from build123d import *

# Parameters (mm, degrees)
F0_R     = 6
F1_DEPTH = 10
F2_R     = 10
F3_DEPTH = 8


with BuildPart() as f1:
    # F0 (on Top) → F1 (new body)
    with BuildSketch(Plane.XY):
        with BuildLine():
            ThreePointArc((-2.287583, -36.367918), (14.118454, -23.224109), (34.477123, -17.985565))
            ThreePointArc((34.477123, -17.985565), (51.756399, 0), (34.477123, 17.985565))
            ThreePointArc((34.477123, 17.985565), (14.118454, 23.224109), (-2.287583, 36.367918))
            ThreePointArc((-2.287583, 36.367918), (-21.61854, 42.178767), (-34.190148, 26.386157))
            Line((-34.190148, 26.386157), (-34.190148, 23.613843))
            Line((-34.190148, 23.613843), (-34.190148, -23.613843))
            Line((-34.190148, -23.613843), (-34.190148, -26.386157))
            ThreePointArc((-34.190148, -26.386157), (-21.61854, -42.178767), (-2.287583, -36.367918))
        make_face()
        with Locations((-16.243601, -25)):
            Circle(F0_R, mode=Mode.SUBTRACT)
        with Locations((33.756399, 0)):
            Circle(F0_R, mode=Mode.SUBTRACT)
        with Locations((-16.243601, 25)):
            Circle(F0_R, mode=Mode.SUBTRACT)
    extrude(amount=F1_DEPTH)

    # F2 (on Front) → F3 (join, symmetric)
    with BuildSketch(Plane.XZ):
        with BuildLine():
            Line((-75.522877, 0), (18.498397, 0))
            Line((18.498397, 0), (18.498397, 10))
            ThreePointArc((18.498397, 10), (-24.010105, 17.449895), (-61.451666, 38.911565))
            ThreePointArc((-61.451666, 38.911565), (-96.211695, 29.481496), (-75.522877, 0))
        make_face()
        with Locations((-75.522877, 22)):
            Circle(F2_R, mode=Mode.SUBTRACT)
    extrude(amount=F3_DEPTH, both=True)


solid = f1.part
Input: part model. Units: mm. Frame: model coordinates. A direction names the side the tool comes from. Give positions to 0.01 mm unless a question says otherwise; leave off trailing zeros. Order: outer loops, then holes, each group sorted by start corner. A loop starts at its lowest first (then second) coordinate and runs counter-clockwise, first axis right, second up. Notation, with made-up numbers: (34, -5) - (52, -5) arc R16 ccw to (52, 9) - close; hole circle Ø6 at (-37, -36.75). An arc over 180 degrees is marked (long way). Answer as a JSON object with one key per item and string values. Group by question number.
Q1. Line query: probe 1 along Z at (x, y) = (-76, 6.5); probe 2 along Y at (x, z) = (-49, 14.5); probe 3 along X at (y, z) = (-4, 3.5). Output: solid intervals per line, ascending.
Q2. Mould query, pull axis Y, two halves, no side actions, for faces 1 (the face through (-13, -1, 0)), 2 (the face through (-21.9, -42.09, 4.93)), 3 (the face through (14.384, 23.092, 4.93)), 4 (the face through (-10.7, -27.3, 4.9)). Classes: pulls with the +Y half, pulls with the -Y half, needs draft (parallel to the pull), parting line crosses it, or undercut.
Q3. First-contact query: pin 1 Ø12 at (x, z) = (-72.5, 15.5) entering from +Y; pin 2 Ø6 at (y, z) = (-2.5, 25.5) entering from +X; pin 3 Ø7 at (x, y) = (-16.24, -25) entering from +Z; pin 4 Ø19 at (x, y) = (33.76, 0) entering from +Z. Flat tips, straight axial feed; report the tip coordinate or a pass-through.
Q4. Set-up query: faces 5 (the face through (-34.19, 17, 5)), 6 (the face through (-70.1, 0.1, 30.4)), 7 (the face through (-34.19, -17, 5)). Return all of +Z, -Z, +X, -X, +Y, -Y with unobstructed straight access to the full face (end or side cutting, diameter ignored); none if empty.
Q5. Cut plane A-A, the plane y = 0. Output: boundary loops of the cut face in (x, z).
Q6. Cut plane D-D, the plane y = -28.5. Output: boundary loops of the cut face in (x, z).
Q7. Cut plane C-C, the plane z = 17. Output: boundary loops of the cut face in (x, y).
Q8. Cut plane B-B, the plane x = -18. Output: boundary loops of the cut face in (y, z), then the cut area to 3 significant figures.
Results:
{
 "1": {"probe 1": "0.01 to 12.01, 31.99 to 43.99", "probe 2": "-8 to 8", "probe 3": "-87.43 to 29.28, 38.23 to 51.31"},
 "2": {"face 1": "needs draft", "face 2": "pulls with the -Y half", "face 3": "pulls with the +Y half", "face 4": "undercut"},
 "3": {"pin 1": "y = 8", "pin 2": "x = -35.99", "pin 3": "through", "pin 4": "z = 10"},
 "4": {"face 5": "+Z, -Z, -X, +Y", "face 6": "+Y, -Y", "face 7": "+Z, -Z, -X, -Y"},
 "5": {"outline": "(-75.52, 0) - (27.76, 0) - (27.76, 10) - (18.5, 10) arc R125 cw to (-61.45, 38.91) arc R22 ccw (long way) to start; (39.76, 0) - (51.76, 0) - (51.76, 10) - (39.76, 10) - close; hole circle Ø20 at (-75.52, 22)"},
 "6": {"outline": "(-33.9, 0) - (-21.12, 0) - (-21.12, 10) - (-33.9, 10) - close; (-11.37, 0) - (5.75, 0) - (5.75, 10) - (-11.37, 10) - close"},
 "7": {"outline": "(-96.95, -8) - (-84.18, -8) - (-84.18, 8) - (-96.95, 8) - close; (-66.86, -8) - (-22.74, -8) - (-22.74, 8) - (-66.86, 8) - close"},
 "8": {"outline": "(-42.91, 0) - (-30.74, 0) - (-30.74, 10) - (-42.91, 10) - close; (-19.26, 0) - (19.26, 0) - (19.26, 10) - (8, 10) - (8, 15.45) - (-8, 15.45) - (-8, 10) - (-19.26, 10) - close; (30.74, 0) - (42.91, 0) - (42.91, 10) - (30.74, 10) - close", "area": "716 mm^2"}
}
